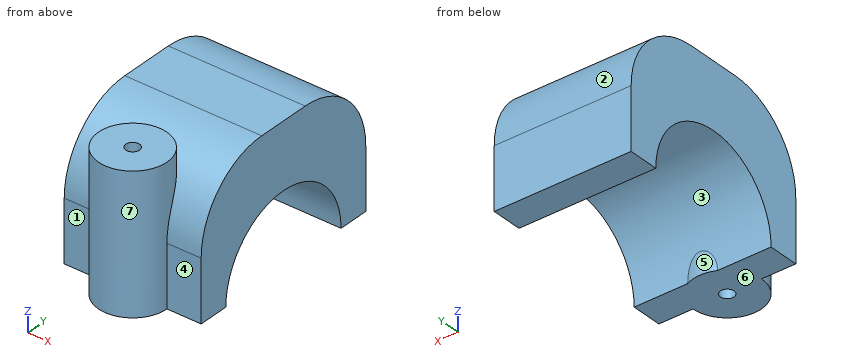
```python
from build123d import *

# Parameters (mm, degrees)
F0_W     = 10
F0_H     = 15
F1_DEPTH = 7.5
F3_DEPTH = 10.001
F4_W     = 10
F4_H     = 15
F5_DEPTH = 2.5
F6_R     = 5.518892
F7_R     = 0.5
F8_DEPTH = 10.001
F7_R_2   = 2.5
F9_DEPTH = 10


with BuildPart() as f1:
    # F0 (on Top) → F1 (new body)
    with BuildSketch(Plane.XY):
        with Locations((5, 7.5)):
            Rectangle(F0_W, F0_H)
    extrude(amount=F1_DEPTH)

    # F2 (on face) → F3 (cut, through all)
    with BuildSketch(Plane(origin=(0, 0, 0), x_dir=(0, -1, 0), z_dir=(-1, 0, 0))):
        with BuildLine():
            Line((-12.75, 0), (-2.25, 0))
            ThreePointArc((-2.25, 0), (-7.5, 5.25), (-12.75, 0))
        make_face()
    extrude(amount=-F3_DEPTH, mode=Mode.SUBTRACT)

    # F4 (on face) → F5 (join)
    with BuildSketch(Plane.XY.offset(7.5)):
        with Locations((5, 7.5)):
            Rectangle(F4_W, F4_H)
    extrude(amount=F5_DEPTH)

    # F6
    f6_edges = [f1.edges().sort_by_distance(p)[0] for p in [
        (5, 15, 10),
        (5, 0, 10),
    ]]
    fillet(f6_edges, radius=F6_R)

    # F7 (on face) → F8 (cut, through all)
    with BuildSketch(Plane.XY.offset(10)):
        with Locations((5, 0)):
            Circle(F7_R)
    extrude(amount=-F8_DEPTH, mode=Mode.SUBTRACT)

    # F7 (on face) → F9 (join)
    with BuildSketch(Plane.XY.offset(10)):
        with Locations((5, 0)):
            Circle(F7_R_2)
        with Locations((5, 0)):
            Circle(F7_R, mode=Mode.SUBTRACT)
    extrude(amount=-F9_DEPTH)


solid = f1.part
```
The listing builds one solid part. Answer for the finished solid, in the listing's coordinates (mm). Face numbers are marked on the shaded views. A direction names the side the tool comes from. Give positions to 0.01 mm unless a question says otherwise; leave off trailing zeros. Write each loop counter-clockwise with the first axis right and the second up, starting at its lowest first coordinate (ties: lowest second). Pieces come first, ordered by that corner, then holes. Notation, with made-up numbers: (78.5, 57.5) - (110.5, 57.5) arc R17 cw to (110.5, 64.5) - close; hole circle Ø7 at (-20, 72.5). An arc over 180 degrees is marked (long way). Use one line per item in the form item = value. Start each with the question number.
1) Find section C-C on z = 5.75. Determine the outline of the cut face in (x, y).
2) The mould has two halves that part along Y. Classify the marked faces 1, 2 and 3: pulls with the +Y half, pulls with the -Y half, needs draft (parallel to the pull), parting line crosses it, or undercut.
3) Find section D-D on y = 7.5. Determine the outline of the cut face in (x, z), plus the area to 3 significant figures.
4) A tool of negligible diameter and unlimited length cuts with its end or side. For the marked faces 4, 5, 6 and 7, from which of +Z, -Z, +X, -X, +Y, -Y can it reach the whole face along a straight path? Write none if from no direction.
5) Find section A-A on z = 1.25. Determine the outline of the cut face in (x, y), plus the area to 3 significant figures.
6) Consider line 1 along Y through (x, z) = (1.5, 0.5); line 2 along Y through (x, z) = (3, 1); line 3 along Y through (x, z) = (7.25, 6.5). Determine where each line is inside the solid, lowest interval first. Write a range as from..to.
7) Find section B-B on x = 8.5. Determine the outline of the cut face in (y, z).
8) Flat-ended cylindrical pins translate along their axes: pin 1 Ø1.5 at (x, y) = (3, 12.5) entering from +Z; pin 2 Ø0.8 at (x, z) = (9, 1.5) entering from -Y; pin 3 Ø1 at (x, y) = (7.5, 11) entering from +Z. Find the tip coordinate at first contact, or state that the pin passes through.
Geometry results:
q1.outline = (0, 0.15) - (2.5, 0.15) arc R2.5 ccw (long way) to (7.5, 0.15) - (10, 0.15) - (10, 14.85) - (0, 14.85) - close; hole circle Ø1 at (5, 0)
q2.face_1 = pulls with the -Y half
q2.face_2 = pulls with the +Y half
q2.face_3 = undercut
q3.outline = (0, 5.25) - (10, 5.25) - (10, 10) - (0, 10) - close
q3.area = 47.5 mm2
q4.face_4 = +Z, -Z, +X, -Y
q4.face_5 = -Z
q4.face_6 = -Z, +X, -X, +Y, -Y
q4.face_7 = +Z
q5.outline = (0, 0) - (2.5, 0) arc R2.5 ccw to (7.5, 0) - (10, 0) - (10, 2.4) - (5.7, 2.4) arc R2.5 ccw to (4.3, 2.4) - (0, 2.4) - close; (0, 12.6) - (10, 12.6) - (10, 15) - (0, 15) - close; hole circle Ø1 at (5, 0)
q5.area = 57.1 mm2
q6.line_1 = 0..2.27, 12.73..15
q6.line_2 = -1.5..2.35, 12.65..15
q6.line_3 = -1.09..14.62
q7.outline = (0, 0) - (2.25, 0) arc R5.25 cw to (12.75, 0) - (15, 0) - (15, 4.48) arc R5.52 ccw to (9.48, 10) - (5.52, 10) arc R5.52 ccw to (0, 4.48) - close
q8.pin_1 = 9.51
q8.pin_2 = 0
q8.pin_3 = 9.91
